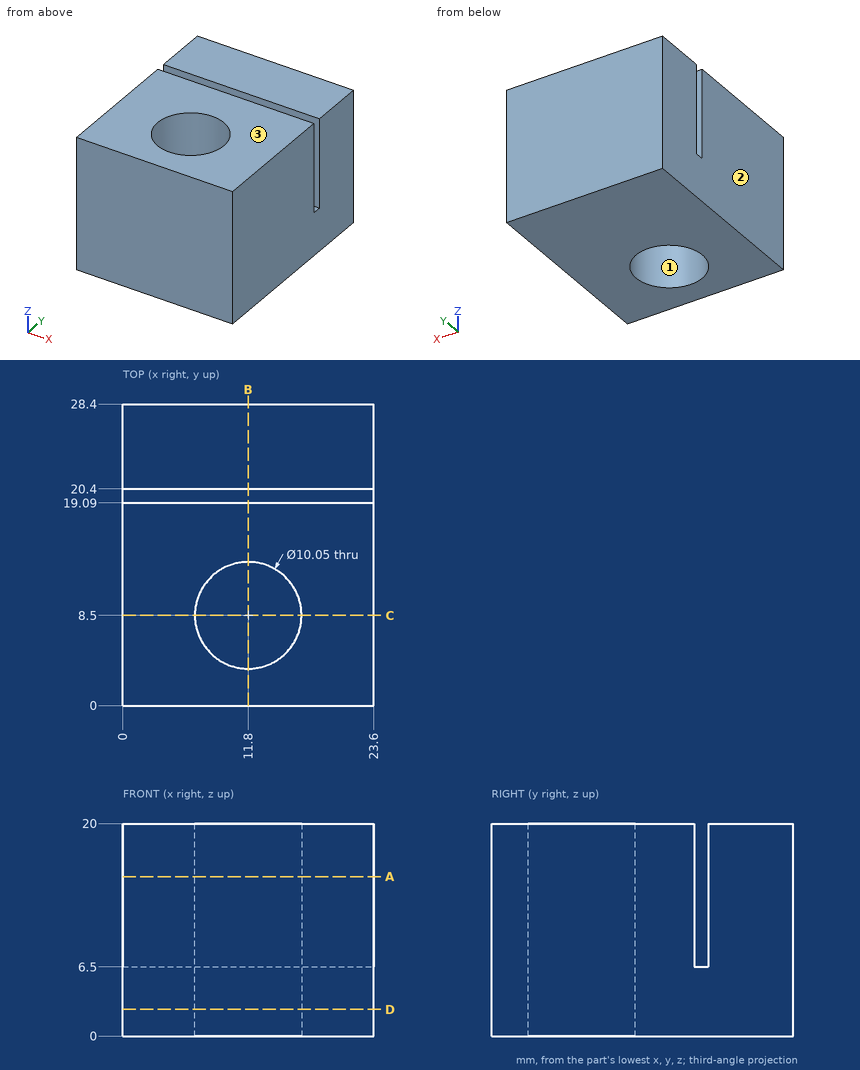
Geometry check sheet. Reference: drawing and pictorial views, mm from the part's lowest x, y, z. Coordinates: 2 decimals unless noted, no trailing zeros. Loops run counter-clockwise (first coordinate to the right, second up) from the corner with the lowest first, then second, coordinate; pieces in that order, holes last.
1) Release check for a two-part mould opening along X. For the marked faces 1, 2 and 3 record: released by +X, released by -X, zero draft, split by the parting line, or undercut.
2) Material ranges on probe 1 along Y at (x, z) = (12, 8.5); probe 2 along Y at (x, z) = (3.75, 14); probe 3 along Y at (x, z) = (13, 17), recorded low to high.
3) Sectioned sample at A-A (z = 15). Record the boundary of the cut face in (x, y) (3 decimals).
4) Sectioned sample at C-C (y = 8.5). Record the boundary of the cut face in (x, z) (3 decimals), and give its area (3 significant figures).
5) Sectioned sample at D-D (z = 2.5). Record the boundary of the cut face in (x, y) (3 decimals).
6) Sectioned sample at B-B (x = 11.8). Record the boundary of the cut face in (y, z) (3 decimals), and give its area (3 significant figures).
7) Gauge pin test, flat end, axial feed: pin 1 (9 mm diameter, centred on x = 11.8, y = 8.5, fed in from -Z). Record the tip position at first contact, or that the pin passes through.
Check sheet entries:
1. face 1: undercut
1. face 2: released by -X
1. face 3: zero draft
2. probe 1: y = 0 to 3.48, 13.52 to 19.09, 20.4 to 28.4
2. probe 2: y = 0 to 19.09, 20.4 to 28.4
2. probe 3: y = 0 to 3.62, 13.38 to 19.09, 20.4 to 28.4
3. outline: (0, 0) - (23.6, 0) - (23.6, 19.09) - (0, 19.09) - close; (0, 20.4) - (23.6, 20.4) - (23.6, 28.4) - (0, 28.4) - close; hole circle Ø10.05 at (11.8, 8.5)
4. outline: (0, 0) - (6.775, 0) - (6.775, 20) - (0, 20) - close; (16.825, 0) - (23.6, 0) - (23.6, 20) - (16.825, 20) - close
4. area: 271 mm2
5. outline: (0, 0) - (23.6, 0) - (23.6, 28.4) - (0, 28.4) - close; hole circle Ø10.05 at (11.8, 8.5)
6. outline: (0, 0) - (3.475, 0) - (3.475, 20) - (0, 20) - close; (13.525, 0) - (28.4, 0) - (28.4, 20) - (20.4, 20) - (20.4, 6.5) - (19.09, 6.5) - (19.09, 20) - (13.525, 20) - close
6. area: 349 mm2
7. pin 1: passes through
